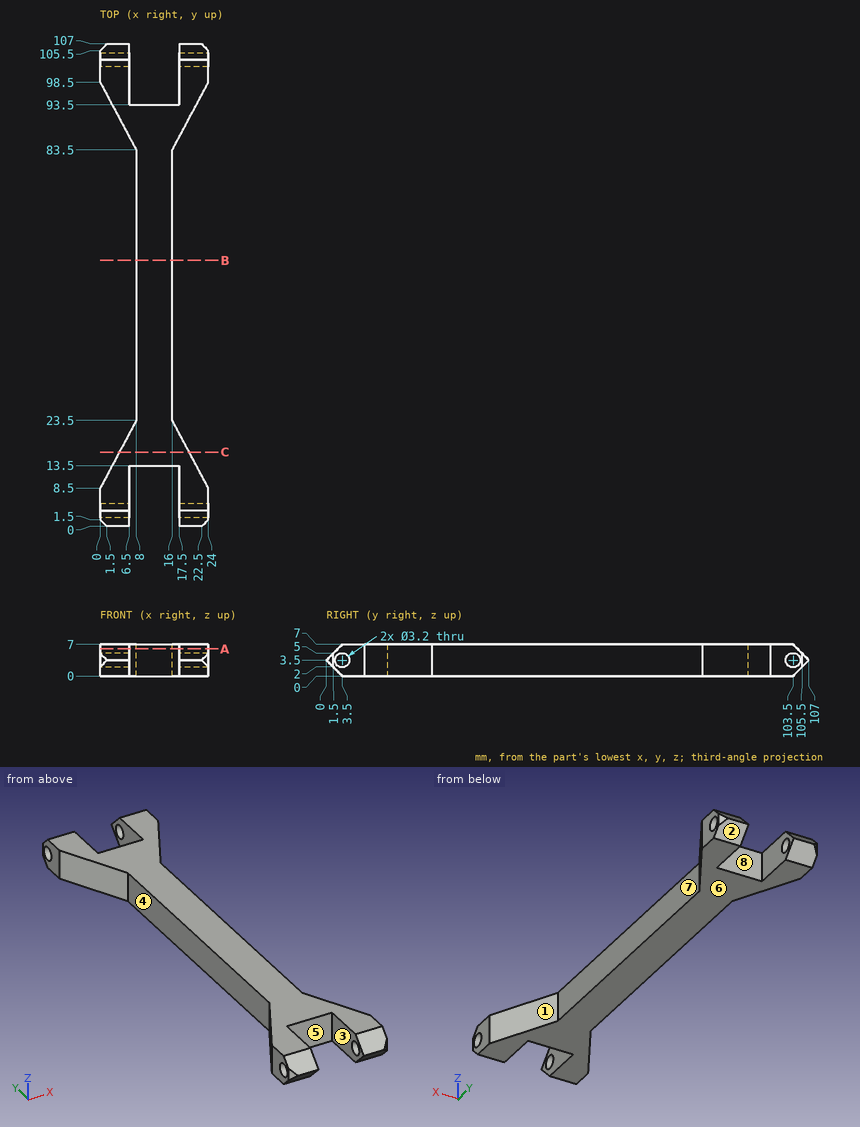
Drawing for the job (mm, zero at the part's lowest x, y, z). A direction names the side the tool comes from. Round coordinates to 2 decimals unless told otherwise and drop trailing zeros. Order: outer loops, then holes, each group sorted by start corner. A loop starts at its lowest first (then second) coordinate and runs counter-clockwise, first axis right, second up. Notation, with made-up numbers: M 6.5,24.5 L 62.5,24.5 A23 cw 62.5,59.5 Z; hole C 58.5,47 d6. An arc over 180 degrees is marked long. Use one line per item in the form item = value.
Q1. Which spindle directions (+Z, -Z, +X, -X, +Y, -Y) get a long thin tool onto all of the face, cutting with end or side? Do the marked faces 4, 5, 6, 7 and 8. Say none if no direction does.
Recorded:
face_4 = +Z, -Z, -X
face_5 = +Z, -Z, -Y
face_6 = -Z, +X, -X, +Y, -Y
face_7 = +Z, -Z, +X
face_8 = +Z, -Z, +Y
Q2. Flat gauge pins, fed straight in: P1, Ø2, axis at y = 63.5, z = 4.5, coming from the -X side; P2, Ø3, axis at y = 72, z = 4.5, coming from the +X side; P3, Ø1, axis at x = 19, z = 2.5, coming from the -Y side; P4, Ø1.9, axis at y = 103.5, z = 3.5, coming from the -X side. Where does each tip first touch, or does it go through?
Recorded:
P1 = 8
P2 = 16
P3 = 0.5
P4 = through
Q3. Saw through at A-A on z = 6. Give the cut face in (x, y).
Recorded:
outline = M 0,2.5 L 6.5,2.5 L 6.5,13.5 L 17.5,13.5 L 17.5,2.5 L 24,2.5 L 24,8.5 L 16,23.5 L 16,83.5 L 24,98.5 L 24,104.5 L 17.5,104.5 L 17.5,93.5 L 6.5,93.5 L 6.5,104.5 L 0,104.5 L 0,98.5 L 8,83.5 L 8,23.5 L 0,8.5 Z
Q4. Saw through at B-B on y = 59. Give the cut face in (x, z).
Recorded:
outline = M 8,0 L 16,0 L 16,7 L 8,7 Z
Q5. Saw through at C-C on y = 16.5. Give the cut face in (x, z), then the cut area to 3 significant figures.
Recorded:
outline = M 4.27,0 L 19.73,0 L 19.73,7 L 4.27,7 Z
area = 108 mm^2
Q6. Two-plate mould, pull along Y, no slides. Class the marked faces 1, 2 and 3: +Y half, -Y half, draft (parallel to the pull), parting line (faces both ways), or undercut.
Recorded:
face_1 = undercut
face_2 = +Y half
face_3 = draft
Q7. Probe L1, parallel to Z at x = 22, y = 3.5; L2, parallel to Z at x = 4.25, y = 103; L3, parallel to X at y = 49.5, z = 4.5. List the from-to ranges inside material, lowest first.
Recorded:
L1 = 0 to 1.9, 5.1 to 7
L2 = 0 to 1.98, 5.02 to 7
L3 = 8 to 16
